The model under review builds one solid part; all positions refer to its coordinate system, in mm. A direction names the side the tool comes from. Coordinates: 2 decimals unless noted, no trailing zeros. Write each loop counter-clockwise with the first axis right and the second up, starting at its lowest first coordinate (ties: lowest second). Pieces come first, ordered by that corner, then holes. Notation, with made-up numbers: (-10, -23.75) - (18, -23.75) arc R14 ccw to (18, -4.75) - close; hole circle Ø8 at (37.5, 70.25). An arc over 180 degrees is marked (long way). Put each result on its own line as item: value.
Autodesk Inventor part; units mm, degrees
ref_plane "YZ Plane" through (0, 0, 0) normal (1, 0, 0) x (0, 1, 0)
ref_plane "XZ Plane" through (0, 0, 0) normal (0, 1, 0) x (-1, 0, 0)
ref_plane "XY Plane" through (0, 0, 0) normal (0, 0, 1) x (1, 0, 0)
sketch "Sketch1" plane through (0, 0, 0) normal (0, 1, 0) x (-1, 0, 0)
  line L0 (22.5, 125) -> (-22.5, 125)
  line L1 (-22.5, 125) -> (-22.5, -125)
  line L2 (-22.5, -125) -> (22.5, -125)
  line L3 (22.5, -125) -> (22.5, 125)
  line L4 (22.5, 125) -> (-22.5, -125) construction
  line L5 (-22.5, 125) -> (22.5, -125) construction
  point P0 (0, 0)
  dimension "d0" = 250
  dimension "d1" = 45
extrude "Extrusion1" add sketch "Sketch1" along normal blind 20
sketch "Sketch2" plane through (0, 0, 0) normal (0, -1, 0) x (1, 0, 0)
  circle A0 centre (0, 100) radius 17.75
  circle A1 centre (0, 50) radius 17.75
  circle A2 centre (0, -50) radius 17.75
  line L0 (0, 50) -> (0, -50) construction
  line L1 (0, 100) -> (0, 50) construction
  line L2 (0, 0) -> (0, 148) construction
  line L3 (-35.7491, 0) -> (26.8031, 0) construction
  line L4 (0, -6) -> (-22.5, -6)
  line L5 (-22.5, -6) -> (-22.5, 6)
  line L6 (-22.5, 6) -> (0, 6)
  line L7 (0, 6) -> (0, -6)
  line L8 (0, -6) -> (-22.5, 6) construction
  line L9 (-22.5, -6) -> (0, 6) construction
  line L10 (-18, 98) -> (-18, -100)
  line L11 (-22.5, 125) -> (22.5, 125)
  line L12 (-22.5, -125) -> (-22.5, 125)
  point P0 (0, 75)
  point P1 (-11.5, 0)
  point P2 (-11.25, 0)
  point P3 (-25, -148)
  point P4 (-16, 100)
  dimension "d9" = 35.5
  dimension "d10" = 35.5
  dimension "d11" = 35.5
  dimension "d12" = 50
  dimension "d13" = 100
  dimension "d16" = 12
  dimension "d36" = 25
sketch "Sketch4" plane through (22.5, 0, 125) normal (1, 0, 0) x (0, 0, -1)
  line L0 (250, 0) -> (230, 20)
  line L1 (0, 20) -> (250, 20)
  line L2 (250, 0) -> (250, 20)
  point P0 (125, 0)
  dimension "d29" = 45
extrude "Extrusion4" cut sketch "Sketch4" against normal through all
extrude "Extrusion5" cut sketch "Sketch2" against normal through all
equation "\"d9\" = d11"
equation "\"d10\" = d11"
equation "\"d13\" = 2 * d12"
properties part number "stand1" material "Wood (Walnut)"
1. Consider section C-C on x = -9. State the section outline as (y, z) points.
Determined:
outline: (0, -125) - (20, -105) - (20, -65.3) - (0, -65.3) - close; (0, -34.7) - (20, -34.7) - (20, -6) - (0, -6) - close; (0, 6) - (20, 6) - (20, 34.7) - (0, 34.7) - close; (0, 65.3) - (20, 65.3) - (20, 84.7) - (0, 84.7) - close; (0, 115.3) - (20, 115.3) - (20, 125) - (0, 125) - close
2. The part is to be moulded in two halves that separate along X. For faces 3 (the flat face through (0, 20, -14)), 4 (the flat face through (22.5, 10, 2)), 5 (the cylindrical face through (-2.3, 9.9, -32.4)), 6 (the cylindrical face through (9.54, 9.86, 64.97)), say which applies: +X half, -X half, draft (parallel to the pull), parting line (faces both ways), or undercut.
Determined:
face 3: draft
face 4: +X half
face 5: undercut
face 6: undercut
3. Consider section A-A on y = 14. State the section outline as (x, z) points.
Determined:
outline: (-22.5, -111) - (22.5, -111) - (22.5, 125) - (-22.5, 125) - (-22.5, 6) - (0, 6) - (0, -6) - (-22.5, -6) - close; hole circle Ø35.5 at (0, -50); hole circle Ø35.5 at (0, 50); hole circle Ø35.5 at (0, 100)
4. To check wall thickness, follow probe 1 along Z at (x, y) = (6, 14.25); probe 2 along Z at (x, y) = (-5, 5); probe 3 along Z at (x, y) = (9, 14). State the ranges of each line that lie inside material, in increasing order.
Determined:
probe 1: z = -110.75 to -66.71, -33.29 to 33.29, 66.71 to 83.29, 116.71 to 125
probe 2: z = -120 to -67.03, -32.97 to -6, 6 to 32.97, 67.03 to 82.97, 117.03 to 125
probe 3: z = -111 to -65.3, -34.7 to 34.7, 65.3 to 84.7, 115.3 to 125
5. Machinability: for faces 1 (the cylindrical face through (-3.848, 9.86, 82.672)), 2 (the flat face through (-11, 10, -6)), which of the approach directions +Z, -Z, +X, -X, +Y, -Y give a long, thin tool a straight path to every point of the face, cutting with its end or side? Answer none if there is none.
Determined:
face 1: +Y, -Y
face 2: -X, +Y, -Y
6. Consider section B-B on z = -50. State the section outline as (x, y) points, plus the area to 3 significant figures.
Determined:
outline: (-22.5, 0) - (-17.75, 0) - (-17.75, 20) - (-22.5, 20) - close; (17.75, 0) - (22.5, 0) - (22.5, 20) - (17.75, 20) - close
area: 190 mm^2
7. For pin 1 Ø6 at (x, y) = (-15.5, 17) entering from -Z; pin 2 Ø1 at (x, y) = (-16.5, 16.5) entering from -Z; pin 3 Ø10 at (x, y) = (-9.5, 13.5) entering from -Z, all flat-tipped, find the tip position at first contact; note any pin that passes through.
Determined:
pin 1: stops at z = -111
pin 2: stops at z = -109
pin 3: stops at z = -116.5
